Can you work these out from the model? Positions are in its coordinate system, mm. A direction names the side the tool comes from. Give positions to 0.01 mm unless a question says otherwise; leave off trailing zeros. Order: outer loops, then holes, each group sorted by start corner. A loop starts at its lowest first (then second) coordinate and runs counter-clockwise, first axis right, second up.
Item 1: If I drill on line 1 along Y through (x, z) = (-5.25, 2.65); line 2 along Z through (x, y) = (-3.25, 2.5); line 3 along Y through (x, z) = (3.25, 1.2), over which ranges is the centre line in solid material (lowest first)?
Item 2: Which directions (+Z, -Z, +X, -X, +Y, -Y) give clear straight access to the entire face, cutting with the end or side of a thin tool? Please do faces 1 (the cylindrical face through (-1.38, -0.91, 1.37)), 2 (the flat face through (-2, 2.3, 2)), 3 (the flat face through (-2, -2.3, 2)).
Item 3: I want a section at D-D, the plane y = 4. Write out the boundary of the cut face in (x, z).
Item 4: I want a section at C-C, the plane z = 1.5. Write out the boundary of the cut face in (x, y).
Item 5: If we mould it in two halves opening along Y, with no side actions, what happens to faces 4 (the flat face through (-1.6, -5, 0.5)), 5 (the cylindrical face through (-1.38, 0.91, 1.37)), 6 (the flat face through (-2, -2, 3)), 7 (the flat face through (-1.6, 5, 0.5))? For each: +Y half, -Y half, draft (parallel to the pull), parting line (faces both ways), or undercut.
Item 6: I want a section at A-A, the plane z = 2.5. Write out the boundary of the cut face in (x, y).
Item 7: I'm going to push flat-ended pins straight in: pin 1 Ø1.4 at (x, y) = (2, 4) entering from +Z; pin 2 Ø0.6 at (x, z) = (2, 2.5) entering from -Y. Where does each tip first touch, or does it pass through?
```python
from build123d import *

# Parameters (mm, degrees)
SKIZZE1_W                       = 17
SKIZZE1_H                       = 10
AUFSATZ_LINEAR_AUSTRAGEN1_DEPTH = 1
SKIZZE2_W                       = 17
SKIZZE2_H                       = 1
AUFSATZ_LINEAR_AUSTRAGEN2_DEPTH = 2
VERRUNDUNG1_R                   = 1.3


with BuildPart() as part:
    # Skizze1 → Aufsatz-Linear austragen1 (new body)
    with BuildSketch(Plane.XY):
        with Locations((-1.5, 0)):
            Rectangle(SKIZZE1_W, SKIZZE1_H)
    extrude(amount=AUFSATZ_LINEAR_AUSTRAGEN1_DEPTH)

    # Skizze2 → Aufsatz-Linear austragen2 (add)
    with BuildSketch(Plane.XY.offset(1)):
        with Locations((-1.5, 1.8)):
            Rectangle(SKIZZE2_W, SKIZZE2_H)
        with Locations((-1.5, -1.8)):
            Rectangle(SKIZZE2_W, SKIZZE2_H)
    extrude(amount=AUFSATZ_LINEAR_AUSTRAGEN2_DEPTH)

    # Verrundung1
    verrundung1_edges = [part.edges().sort_by_distance(p)[0] for p in [
        (-1.5, -1.3, 1),
        (-1.5, 1.3, 1),
    ]]
    fillet(verrundung1_edges, radius=VERRUNDUNG1_R - 0.0001)  # a hair under: the kernel refuses the full size


solid = part.part
```
Results list:
1. line 1: y = -2.3 to -1.3, 1.3 to 2.3
1. line 2: z = 0 to 1
1. line 3: y = -2.3 to -0.69, 0.69 to 2.3
2. face 1: +Z, +X, -X
2. face 2: +Z, +X, -X, +Y
2. face 3: +Z, +X, -X, -Y
3. outline: (-10, 0) - (7, 0) - (7, 1) - (-10, 1) - close
4. outline: (-10, -2.3) - (7, -2.3) - (7, -1.02) - (-10, -1.02) - close; (-10, 1.02) - (7, 1.02) - (7, 2.3) - (-10, 2.3) - close
5. face 4: -Y half
5. face 5: undercut
5. face 6: draft
5. face 7: +Y half
6. outline: (-10, -2.3) - (7, -2.3) - (7, -1.3) - (-10, -1.3) - close; (-10, 1.3) - (7, 1.3) - (7, 2.3) - (-10, 2.3) - close
7. pin 1: stops at z = 1
7. pin 2: stops at y = -2.3
